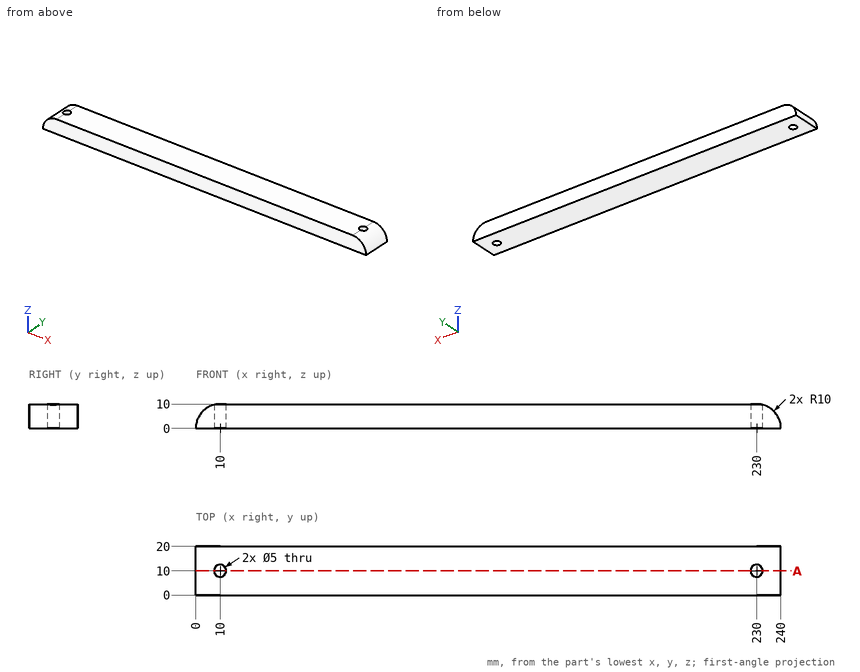
Answer from the drawing. Dimensions are ordinates in mm from the lowest x, y and z of the part. Give positions to 0.01 mm unless a question says otherwise; leave off trailing zeros. Write each loop counter-clockwise with the first axis right and the second up, starting at its lowest first coordinate (ties: lowest second). Pieces come first, ordered by that corner, then holes.
1) Find the intervals of material crossed by L1, parallel to X at y = 12, z = 5; L2, parallel to Y at x = 230, z = 6.25; L3, parallel to X at y = 8.75, z = 6.25, in increasing order.
2) Section A-A (y = 10) is taken. Write down the section's boundary in (x, z), and give its area (3 significant figures).
3) Given P1, Ø2, axis at y = 10.5, z = 8, coming from the -X side; P2, Ø1.5, axis at y = 13.5, z = 4, coming from the -X side; P3, Ø4.5, axis at x = 230, y = 10, coming from the +Z side, each flat-ended and moving along its own axis, determine where each tip first touches the part or whether it passes through.
Response:
1. L1: x = 1.34 to 8.5, 11.5 to 228.5, 231.5 to 238.66
1. L2: y = 0 to 7.5, 12.5 to 20
1. L3: x = 2.19 to 7.83, 12.17 to 227.83, 232.17 to 237.81
2. outline: (0, 0) - (7.5, 0) - (7.5, 9.68) arc R10 ccw to start; (12.5, 0) - (227.5, 0) - (227.5, 10) - (12.5, 10) - close; (232.5, 0) - (240, 0) arc R10 ccw to (232.5, 9.68) - close
2. area: 2,260 mm2
3. P1: stops at x = 2.86
3. P2: stops at x = 0.54
3. P3: passes through
